For this review, take the finished solid that the model builds, in its own axes (mm). Coordinates: 2 decimals unless noted, no trailing zeros. Loops run counter-clockwise (first coordinate to the right, second up) from the corner with the lowest first, then second, coordinate; pieces in that order, holes last. Notation, with made-up numbers: (50, 50.5) -> (64, 50.5) arc R9 cw to (64, 60.5) -> close; hole circle Ø10 at (15, -3). An arc over 180 degrees is marked (long way). Use a Markdown table: item, result.
Autodesk Inventor part; units mm, degrees
ref_plane "YZ Plane" through (0, 0, 0) normal (1, 0, 0) x (0, 1, 0)
ref_plane "XZ Plane" through (0, 0, 0) normal (0, 1, 0) x (-1, 0, 0)
ref_plane "XY Plane" through (0, 0, 0) normal (0, 0, 1) x (1, 0, 0)
sketch "Sketch1" plane through (0, 0, 0) normal (0, 1, 0) x (-1, 0, 0)
  line L0 (-56.25, 58.25) -> (56.25, 58.25)
  line L1 (56.25, 58.25) -> (56.25, -58.25)
  line L2 (56.25, -58.25) -> (-56.25, -58.25)
  line L3 (-56.25, -58.25) -> (-56.25, 58.25)
  line L4 (-56.25, 58.25) -> (56.25, -58.25) construction
  line L5 (56.25, 58.25) -> (-56.25, -58.25) construction
  point P0 (0, 0)
  dimension "d0" = 112.5
  dimension "d1" = 116.5
extrude "Extrusion1" add sketch "Sketch1" along normal blind 5
sketch "Sketch2" plane through (0, 5, 0) normal (0, 1, 0) x (1, 0, 0)
  circle A0 centre (18.5, 27.9796) radius 23.85
  circle A1 centre (37, -23.25) radius 13.85
  circle A2 centre (-35, -40.25) radius 13.85
  circle A3 centre (-30.9, 25.8198) radius 13.85
  circle A4 centre (0, -23.25) radius 13.85
  line L0 (56.25, 58.25) -> (-56.25, 58.25)
  line L1 (-56.25, -58.25) -> (56.25, -58.25)
  line L2 (0, -105.9299) -> (0, 123.2086) construction
  line L3 (-76.4777, -40.25) -> (-5.35, -40.25) construction
  line L4 (-123.5447, -23.25) -> (82.5572, -23.25) construction
  line L5 (56.25, -58.25) -> (56.25, 58.25) construction
  point P0 (0, 0)
  dimension "d4" = 47.7
  dimension "d5" = 27.7
  dimension "d6" = 27.7
  dimension "d7" = 27.7
  dimension "d8" = 27.7
  dimension "d9" = 116.5
  dimension "d10" = 112.5
  dimension "d13" = 37
  dimension "d14" = 18.5
  dimension "d15" = 30.9
  dimension "d18" = 18
  dimension "d19" = 35
  dimension "d20" = 35
extrude "Extrusion2" cut sketch "Sketch2" against normal blind 5
properties part number "Bottle layout lower plate"
(1) Take a section at A-A on z = 23.25. Write out the cut boundary in (x, y), plus the area to 4 significant figures.
Found:
| item | result |
|---|---|
| outline | (-56.25, 0) -> (-13.85, 0) -> (-13.85, 5) -> (-56.25, 5) -> close; (13.85, 0) -> (23.15, 0) -> (23.15, 5) -> (13.85, 5) -> close; (50.85, 0) -> (56.25, 0) -> (56.25, 5) -> (50.85, 5) -> close |
| area | 285.5 mm^2 |
(2) For pin 1 Ø16.5 at (x, z) = (37, 23.25) entering from +Y, flat-tipped, find the tip position at first contact; note if it passes through.
Found:
| item | result |
|---|---|
| pin 1 | passes through |
(3) Mouldability with a two-part tool opening along X and no side actions: class faces 1 (the face through (1, 2, 58.25)), 2 (the face through (0.922, 2.535, -44.099)), 3 (the face through (-56.25, 2, 1)), 4 (the face through (56.25, 2, -1)) as pulls with the +X half, pulls with the -X half, needs draft (parallel to the pull), parting line crosses it, or undercut.
Found:
| item | result |
|---|---|
| face 1 | needs draft |
| face 2 | undercut |
| face 3 | pulls with the -X half |
| face 4 | pulls with the +X half |
(4) Take a section at D-D on z = 40.25. Write out the cut boundary in (x, y).
Found:
| item | result |
|---|---|
| outline | (-56.25, 0) -> (-48.85, 0) -> (-48.85, 5) -> (-56.25, 5) -> close; (-21.15, 0) -> (56.25, 0) -> (56.25, 5) -> (-21.15, 5) -> close |
(5) Take a section at B-B on x = -19. Write out the cut boundary in (y, z).
Found:
| item | result |
|---|---|
| outline | (0, -58.25) -> (5, -58.25) -> (5, -32.91) -> (0, -32.91) -> close; (0, -18.73) -> (5, -18.73) -> (5, 58.25) -> (0, 58.25) -> close |
(6) Take a section at C-C on x = -35. Write out the cut boundary in (y, z).
Found:
| item | result |
|---|---|
| outline | (0, -58.25) -> (5, -58.25) -> (5, -39.05) -> (0, -39.05) -> close; (0, -12.59) -> (5, -12.59) -> (5, 26.4) -> (0, 26.4) -> close; (0, 54.1) -> (5, 54.1) -> (5, 58.25) -> (0, 58.25) -> close |
(7) For line 1 along X through (y, z) = (2.9, 23.25); line 2 along Z through (x, y) = (18.5, 3.9); line 3 along X through (y, z) = (3.35, 40.25), list the stretches that pass through material, from the lowest coordinate up.
Found:
| item | result |
|---|---|
| line 1 | x = -56.25 to -13.85, 13.85 to 23.15, 50.85 to 56.25 |
| line 2 | z = -58.25 to -51.83, -4.13 to 58.25 |
| line 3 | x = -56.25 to -48.85, -21.15 to 56.25 |
